Input: part model. Units: mm. Frame: model coordinates. A direction names the side the tool comes from. Give positions to 0.01 mm unless a question says otherwise; leave off trailing zeros. Write each loop counter-clockwise with the first axis right and the second up, starting at its lowest first coordinate (ties: lowest second). Pieces come first, ordered by that corner, then holes. Notation, with made-up numbers: (-8, 54) -> (33, 54) arc R19 ccw to (33, 83) -> close; hole circle Ø11 at (18, 64). An arc over 180 degrees is marked (long way). Answer as a JSON object with one key per item and string values. Group by question number.
from build123d import *

# Parameters (mm, degrees)
SKETCH1_R           = 20
BOSS_EXTRUDE1_DEPTH = 40
SKETCH2_R           = 15
BOSS_EXTRUDE2_DEPTH = 30
SKETCH3_R           = 15
BOSS_EXTRUDE3_DEPTH = 30
SKETCH4_R           = 20
SKETCH4_R_2         = 15
CUT_EXTRUDE1_DEPTH  = 15
SKETCH5_W           = 6
SKETCH5_H           = 8
CUT_EXTRUDE2_DEPTH  = 45


with BuildPart() as part:
    # Sketch1 → Boss-Extrude1 (new body, symmetric)
    with BuildSketch(Plane(origin=(0, 0, 0), x_dir=(1, 0, 0), z_dir=(0, 1, 0))):
        Circle(SKETCH1_R)
    extrude(amount=BOSS_EXTRUDE1_DEPTH, both=True)

    # Sketch2 → Boss-Extrude2 (add)
    with BuildSketch(Plane(origin=(0, 40, 0), x_dir=(1, 0, 0), z_dir=(0, 1, 0))):
        Circle(SKETCH2_R)
    extrude(amount=BOSS_EXTRUDE2_DEPTH)

    # Sketch3 → Boss-Extrude3 (add)
    with BuildSketch(Plane.XZ.offset(40)):
        Circle(SKETCH3_R)
    extrude(amount=BOSS_EXTRUDE3_DEPTH)

    # Sketch4 → Cut-Extrude1 (cut)
    with BuildSketch(Plane(origin=(0, 40, 0), x_dir=(1, 0, 0), z_dir=(0, 1, 0))):
        Circle(SKETCH4_R)
        Circle(SKETCH4_R_2, mode=Mode.SUBTRACT)
    extrude(amount=-CUT_EXTRUDE1_DEPTH, mode=Mode.SUBTRACT)

    # Sketch5 → Cut-Extrude2 (cut)
    with BuildSketch(Plane(origin=(0, 70, 0), x_dir=(1, 0, 0), z_dir=(0, 1, 0))):
        with Locations((0, 15)):
            Rectangle(SKETCH5_W, SKETCH5_H)
    extrude(amount=-CUT_EXTRUDE2_DEPTH, mode=Mode.SUBTRACT)


solid = part.part
1. Contact query for flat-ended pins moving along their axis: pin 1 Ø12 at (x, y) = (13, 41.5) entering from +Z; pin 2 Ø1.5 at (x, y) = (11, -44) entering from -Z; pin 3 Ø4 at (y, z) = (50, -13) entering from +X. Output: stop coordinate, or through.
2. Section B-B (z = 0). Return the cut outline in (x, y).
3. Line query: line 1 (Y direction, x = 1.5, z = -15); line 2 (X direction, y = -3.5, z = -1); line 3 (Z direction, x = -0.5, y = -36.5). Output: solid intervals per line, ascending.
4. Section C-C (y = 20.5). Return the cut outline in (x, z).
5. Reachability of faces 4 (the face through (0, 48, -11)), 5 (the face through (3, -40, -15)), 6 (the face through (-4.336, -7.045, 19.524)) from +Z, -Z, +X, -X, +Y, -Y: full face, straight path, thin tool, end or side. Return the list, or none.
6. Section A-A (x = -12). Return the cut outline in (y, z), plus the area to 3 significant figures.
7. Mould query, pull axis X, two halves, no side actions, for faces 1 (the face through (-3, 48, -13)), 2 (the face through (0, 70, 0)), 3 (the face through (-0.617, 47.815, 14.987)). Classes: pulls with the +X half, pulls with the -X half, needs draft (parallel to the pull), parting line crosses it, or undercut.
8. Section D-D (y = 34.5). Return the cut outline in (x, z), plus the area to 3 significant figures.
Working result:
{
 "1": {"pin 1": "stops at z = 13.27", "pin 2": "stops at z = -10.95", "pin 3": "stops at x = 10.2"},
 "2": {"outline": "(-20, -40) -> (-15, -40) -> (-15, -70) -> (15, -70) -> (15, -40) -> (20, -40) -> (20, 25) -> (15, 25) -> (15, 70) -> (-15, 70) -> (-15, 25) -> (-20, 25) -> close"},
 "3": {"line 1": "y = -40 to 25", "line 2": "x = -19.97 to 19.97", "line 3": "z = -19.99 to 19.99"},
 "4": {"outline": "circle Ø40 at (0, 0)"},
 "5": {"face 4": "-Z, +Y", "face 5": "-Y", "face 6": "+Y, -Y"},
 "6": {"outline": "(-70, -9) -> (-40, -9) -> (-40, -16) -> (25, -16) -> (25, -9) -> (70, -9) -> (70, 9) -> (25, 9) -> (25, 16) -> (-40, 16) -> (-40, 9) -> (-70, 9) -> close", "area": "3,430 mm^2"},
 "7": {"face 1": "undercut", "face 2": "needs draft", "face 3": "parting line crosses it"},
 "8": {"outline": "(-3, -14.7) -> (-3, -11) -> (3, -11) -> (3, -14.7) arc R15 ccw (long way) to start", "area": "683 mm^2"}
}
